For this review, use the dimensioned drawing (mm, ordinates from the lowest corner) and the shaded views. A direction names the side the tool comes from. Give positions to 0.01 mm unless a question says otherwise; leave off trailing zeros. Loops run counter-clockwise (first coordinate to the right, second up) from the corner with the lowest first, then second, coordinate; pieces in that order, holes last. Notation, with made-up numbers: M -23.5,28.25 L -19.5,28.25 A31 ccw -19.5,54.25 Z; hole C 80,59 d9. An arc over 180 degrees is marked long. Return JSON: item names as keys, results as strings.
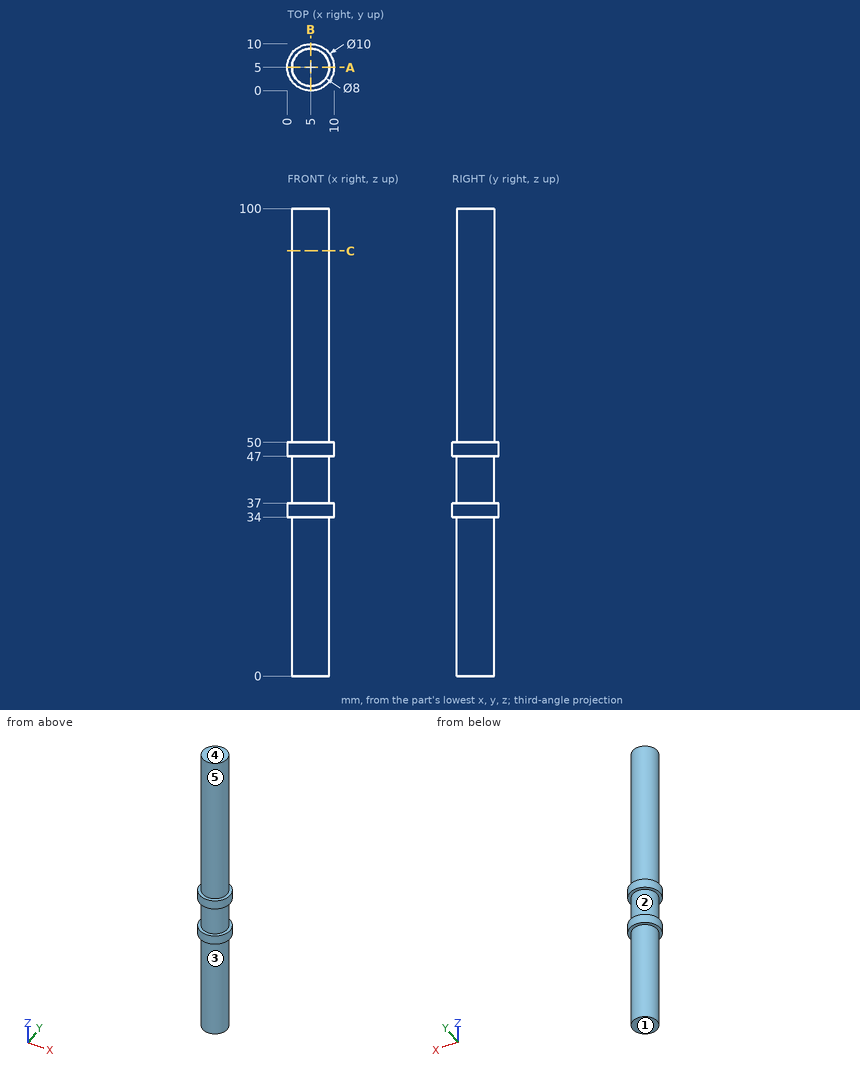
1) Consider section A-A on y = 5. Write out the cut boundary in (x, z), then the cut area to 3 significant figures.
From the geometry:
{"outline": "M 0,34 L 1,34 L 1,0 L 9,0 L 9,34 L 10,34 L 10,37 L 9,37 L 9,47 L 10,47 L 10,50 L 9,50 L 9,100 L 1,100 L 1,50 L 0,50 L 0,47 L 1,47 L 1,37 L 0,37 Z", "area": "812 mm²"}
2) Consider section C-C on z = 91. Write out the cut boundary in (x, y), then the cut area to 3 significant figures.
From the geometry:
{"outline": "C 5,5 d8", "area": "50.3 mm²"}
3) Tool access review of the marked faces 1, 2, 3, 4 and 5: name each direction out of +Z, -Z, +X, -X, +Y, -Y from which nothing blocks a thin tool from reaching the whole face with its end or side.
From the geometry:
{"face 1": "-Z, +X, -X, +Y, -Y", "face 2": "none", "face 3": "-Z", "face 4": "+Z, +X, -X, +Y, -Y", "face 5": "+Z"}
4) Insertion check: pin 1 (4 mm diameter, centred on x = 6.5, z = 54.5, fed in from -Y); pin 2 (6 mm diameter, centred on y = 8, z = 84, fed in from +X); pin 3 (2 mm diameter, centred on y = 1.5, z = 78.5, fed in from +X). Each pin has a flat end and moves straight along its axis. Give the tip position at first contact, or say it passes through.
From the geometry:
{"pin 1": "y = 1", "pin 2": "x = 9", "pin 3": "x = 8.12"}
5) Wall thickness on L1, parallel to Z at x = 1, y = 7.25; L2, parallel to X at y = 5.5, z = 19; L3, parallel to Y at x = 8, z = 57: over which ranges is each line inside the solid? List them lowest first. Write a range as from..to.
From the geometry:
{"L1": "34..37, 47..50", "L2": "1.03..8.97", "L3": "2.35..7.65"}
